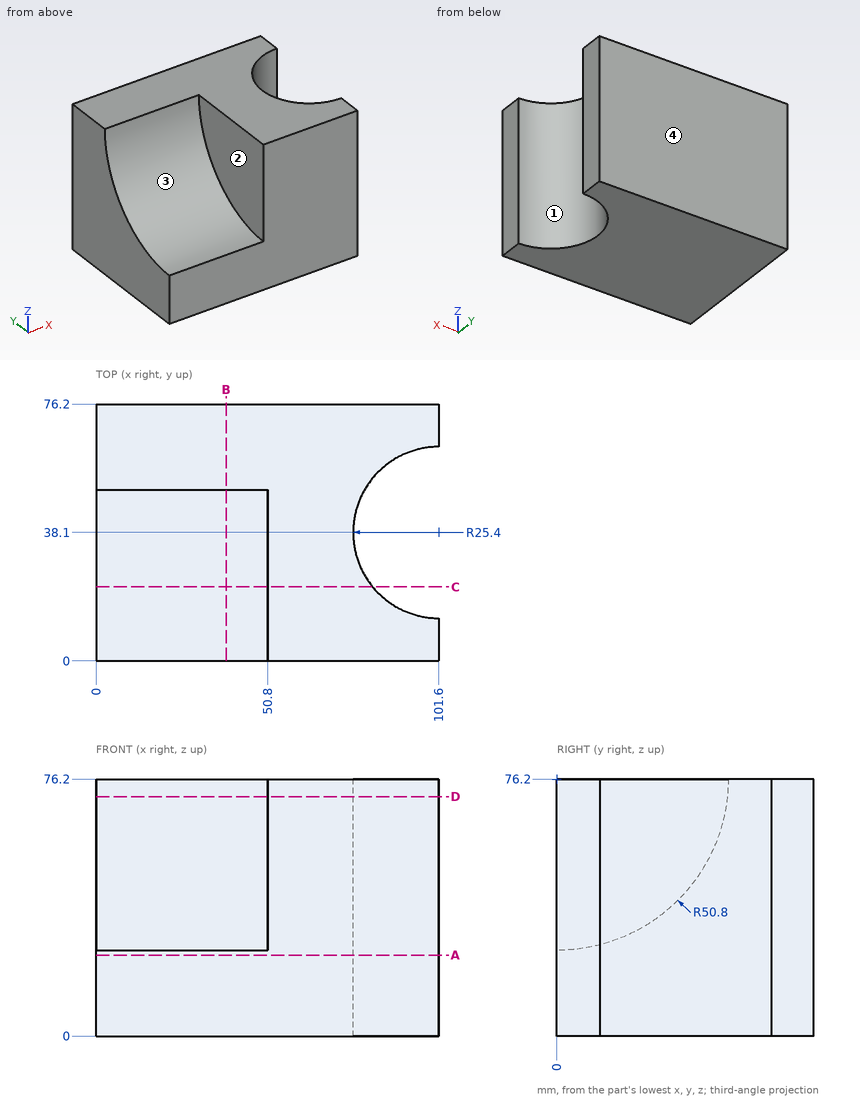
Here's the drawing with two shaded views (mm, measured from the low corner). I have some questions. Coordinates: 2 decimals unless noted, no trailing zeros. Loops run counter-clockwise (first coordinate to the right, second up) from the corner with the lowest first, then second, coordinate; pieces in that order, holes last. Notation, with made-up numbers: (62, 61) -> (115, 61) arc R32 ccw to (115, 88) -> close; hole circle Ø4 at (17.5, 16.25). An arc over 180 degrees is marked (long way). Answer in a Markdown table with one row per item.
(1) Thinking about a two-plate mould opening in Y: for the marked faces 1, 2, 3 and 4, which applies, released by +Y, released by -Y, zero draft, split by the parting line, or undercut?
Results found:
| item | result |
|---|---|
| face 1 | undercut |
| face 2 | zero draft |
| face 3 | released by -Y |
| face 4 | released by +Y |
(2) Imagine slicing it at C-C (y = 22). List the corners of the cut face in (x, z) for me.
Results found:
| item | result |
|---|---|
| outline | (0, 0) -> (81.95, 0) -> (81.95, 76.2) -> (50.8, 76.2) -> (50.8, 30.41) -> (0, 30.41) -> close |
(3) Imagine slicing it at A-A (z = 24). List the corners of the cut face in (x, y) for me.
Results found:
| item | result |
|---|---|
| outline | (0, 0) -> (101.6, 0) -> (101.6, 12.7) arc R25.4 cw to (101.6, 63.5) -> (101.6, 76.2) -> (0, 76.2) -> close |
(4) Imagine slicing it at D-D (z = 71). List the corners of the cut face in (x, y) for me.
Results found:
| item | result |
|---|---|
| outline | (0, 50.53) -> (50.8, 50.53) -> (50.8, 0) -> (101.6, 0) -> (101.6, 12.7) arc R25.4 cw to (101.6, 63.5) -> (101.6, 76.2) -> (0, 76.2) -> close |
(5) If I drill on probe 1 along X at (y, z) = (39, 17); probe 2 along X at (y, z) = (5.5, 57.5); probe 3 along Y at (x, z) = (96.5, 43), over which ranges is the centre line in solid material (lowest first)?
Results found:
| item | result |
|---|---|
| probe 1 | x = 0 to 76.22 |
| probe 2 | x = 50.8 to 101.6 |
| probe 3 | y = 0 to 13.22, 62.98 to 76.2 |
(6) Will this pin go through, and if not, where does the flat tip stop? pin 1 Ø4 at (y, z) = (24, 35) entering from -X.
Results found:
| item | result |
|---|---|
| pin 1 | stops at x = 50.8 |
(7) Imagine slicing it at B-B (x = 38.5). List the corners of the cut face in (y, z) for me.
Results found:
| item | result |
|---|---|
| outline | (0, 0) -> (76.2, 0) -> (76.2, 76.2) -> (50.8, 76.2) arc R50.8 cw to (0, 25.4) -> close |
